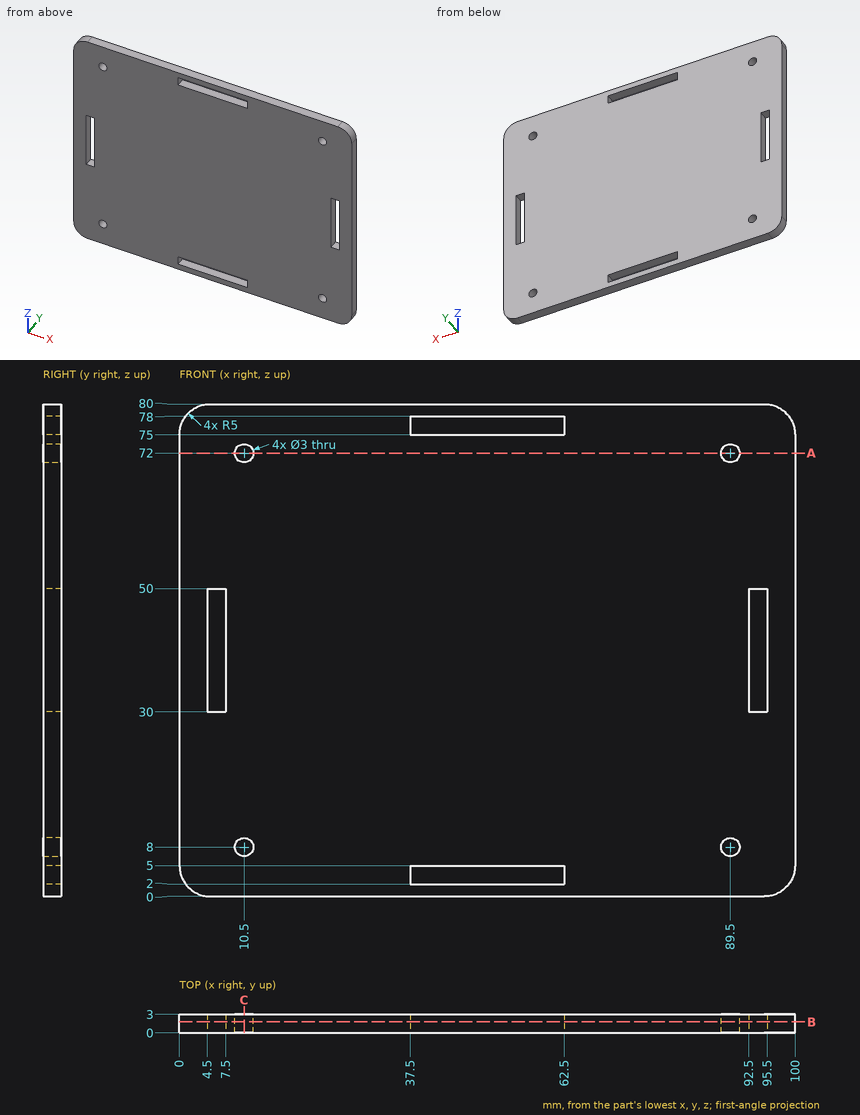
Design review of the part shown in the three views and the two pictorial views. Dimensions are in mm from the part's minimum x, y and z. Round coordinates to 2 decimals unless told otherwise and drop trailing zeros. Write each loop counter-clockwise with the first axis right and the second up, starting at its lowest first coordinate (ties: lowest second). Pieces come first, ordered by that corner, then holes. Notation, with made-up numbers: (41, -24.5) -> (55, -24.5) arc R25 ccw to (55, -1.5) -> close; hole circle Ø6 at (20, 50). An arc over 180 degrees is marked (long way). Write item = value, one per line. Start each with the question number.
1) Take a section at C-C, the plane x = 10.5. State the section outline as (y, z) points, plus the area to 3 significant figures.
2) Clearance check with flat-ended pins moving along their axes: pin 1 (1.5 mm diameter, centred on y = 1.5, z = 3, fed in from +X); pin 2 (0.9 mm diameter, centred on y = 1, z = 77, fed in from -X); pin 3 (2.5 mm diameter, centred on x = 10.5, z = 72, fed in from +Y). State where each tip first meets the part, or that it passes through.
3) Wall thickness on probe 1 along X at (y, z) = (0.35, 41); probe 2 along Z at (x, y) = (89.5, 1.05); probe 3 along Z at (x, y) = (44, 1.5): over which ranges is each line inside the solid? List them lowest first. Write a range as from..to.
4) Take a section at A-A, the plane z = 72. State the section outline as (x, y) points, plus the area to 3 significant figures.
5) Take a section at B-B, the plane y = 1.8. Count the separate pieces of the cut face and the enclosed holes in it, plus the area to 3 significant figures.
Results list:
q1.outline = (0, 0) -> (3, 0) -> (3, 6.5) -> (0, 6.5) -> close; (0, 9.5) -> (3, 9.5) -> (3, 70.5) -> (0, 70.5) -> close; (0, 73.5) -> (3, 73.5) -> (3, 80) -> (0, 80) -> close
q1.area = 222 mm²
q2.pin_1 = 99.84
q2.pin_2 = 0.25
q2.pin_3 = through
q3.probe_1 = 0..4.5, 7.5..92.5, 95.5..100
q3.probe_2 = 0..6.5, 9.5..70.5, 73.5..80
q3.probe_3 = 0..2, 5..75, 78..80
q4.outline = (0, 0) -> (9, 0) -> (9, 3) -> (0, 3) -> close; (12, 0) -> (88, 0) -> (88, 3) -> (12, 3) -> close; (91, 0) -> (100, 0) -> (100, 3) -> (91, 3) -> close
q4.area = 282 mm²
q5.separate_pieces = 1
q5.enclosed_holes = 8
q5.area = 7,680 mm²
